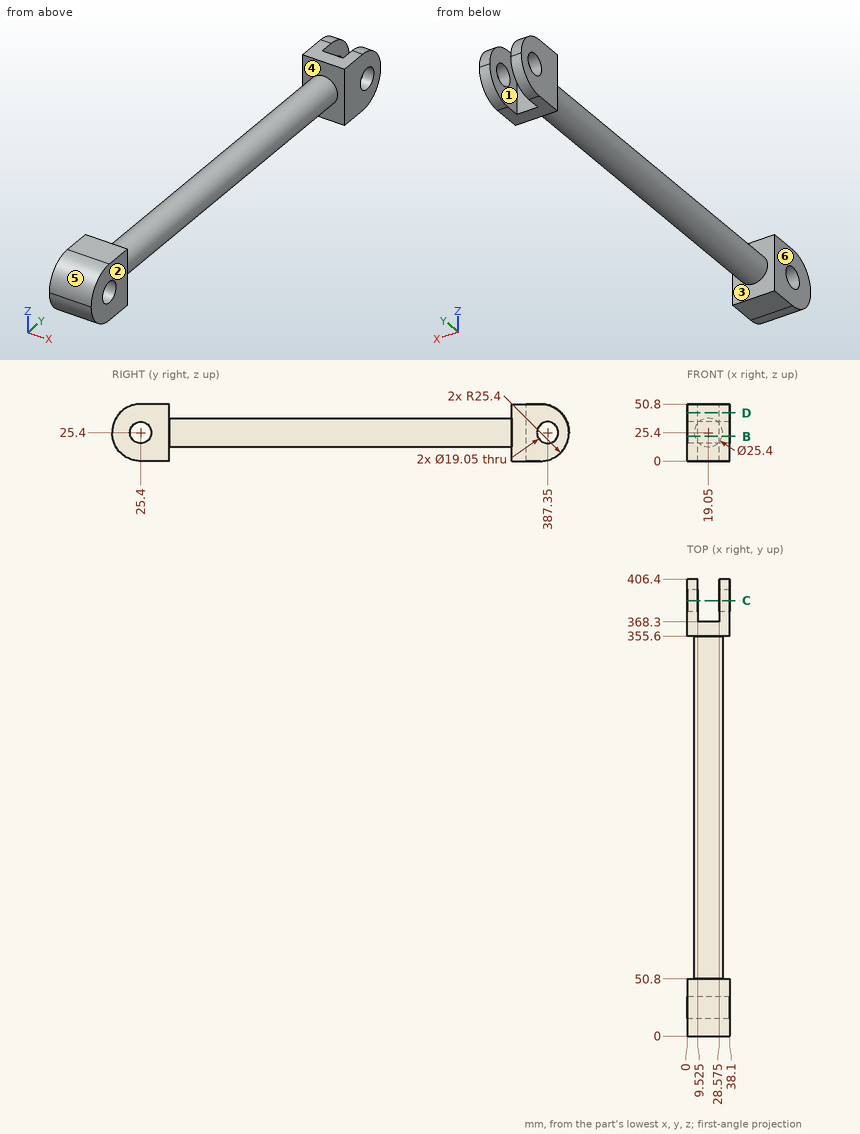
Here's the drawing with two shaded views (mm, measured from the low corner). I have some questions. A direction names the side the tool comes from. Give positions to 0.01 mm unless a question says otherwise; leave off trailing zeros. Order: outer loops, then holes, each group sorted by start corner. A loop starts at its lowest first (then second) coordinate and runs counter-clockwise, first axis right, second up. Notation, with made-up numbers: (-4.75, 40) -> (3.25, 40) arc R19 cw to (3.25, 76) -> close; hole circle Ø9 at (28.25, -35). An arc over 180 degrees is marked (long way). Use a Markdown table: item, result. Add a question column.
Item 1: Imagine slicing it at B-B on z = 22. Please give me the cut outline in (x, y) (1 decimal), plus the area to 3 significant figures.
Item 2: Will these pins go through, and if not, where does the flat tip stop? pin 1 (1.5 mm diameter, centred on y = 272.5, z = 14.5, fed in from +X); pin 2 (15 mm diameter, centred on x = 23, z = 34, fed in from +Y); pin 3 (1.5 mm diameter, centred on x = 27.5, z = 45.5, fed in from +Y).
Item 3: I need wall thicknesses on line 1 (Y direction, x = 7, z = 25); line 2 (Z direction, x = 19.5, y = 25.4) (3 decimals); line 3 (Y direction, x = 21, z = 25). Which ranges of each line are inside material? Lowest first, please.
Item 4: If we mould it in two halves opening along Y, with no side actions, what happens to the marked faces 4, 5 and 6? For each: pulls with the +Y half, pulls with the -Y half, needs draft (parallel to the pull), parting line crosses it, or undercut.
Item 5: Imagine slicing it at D-D on z = 43. Please give me the cut outline in (x, y) (3 decimals), plus the area to 3 significant figures.
Item 6: Imagine slicing it at C-C on y = 387.35. Please give me the cut outline in (x, z) (3 decimals), plus the area to 3 significant figures.
Item 7: For the marked faces 1, 2 and 3, which set-ups out of +Z, -Z, +X, -X, +Y, -Y let a thin tool reach every point of the face, with its end or its side?
Data:
| question | item | result |
|---|---|---|
| 1 | outline | (0, 0.2) -> (38.1, 0.2) -> (38.1, 16.5) -> (0, 16.5) -> close; (0, 34.3) -> (38.1, 34.3) -> (38.1, 50.8) -> (31.3, 50.8) -> (31.3, 355.6) -> (38.1, 355.6) -> (38.1, 378.5) -> (28.6, 378.5) -> (28.6, 368.3) -> (9.5, 368.3) -> (9.5, 378.5) -> (0, 378.5) -> (0, 355.6) -> (6.8, 355.6) -> (6.8, 50.8) -> (0, 50.8) -> close; (0, 396.2) -> (9.5, 396.2) -> (9.5, 406.2) -> (0, 406.2) -> close; (28.6, 396.2) -> (38.1, 396.2) -> (38.1, 406.2) -> (28.6, 406.2) -> close |
| 1 | area | 9,570 mm² |
| 2 | pin 1 | stops at x = 26.68 |
| 2 | pin 2 | stops at y = 406.15 |
| 2 | pin 3 | stops at y = 368.3 |
| 3 | line 1 | y = 0 to 15.88, 34.92 to 377.83, 396.87 to 406.4 |
| 3 | line 2 | z = 0 to 15.875, 34.925 to 50.8 |
| 3 | line 3 | y = 0 to 15.88, 34.92 to 368.3 |
| 4 | face 4 | undercut |
| 4 | face 5 | pulls with the -Y half |
| 4 | face 6 | needs draft |
| 5 | outline | (0, 7.086) -> (38.1, 7.086) -> (38.1, 50.8) -> (0, 50.8) -> close; (0, 355.6) -> (38.1, 355.6) -> (38.1, 399.314) -> (28.575, 399.314) -> (28.575, 368.3) -> (9.525, 368.3) -> (9.525, 399.314) -> (0, 399.314) -> close |
| 5 | area | 2,740 mm² |
| 6 | outline | (0, 0.807) -> (9.525, 0.807) -> (9.525, 15.875) -> (0, 15.875) -> close; (0, 34.925) -> (9.525, 34.925) -> (9.525, 49.993) -> (0, 49.993) -> close; (28.575, 0.807) -> (38.1, 0.807) -> (38.1, 15.875) -> (28.575, 15.875) -> close; (28.575, 34.925) -> (38.1, 34.925) -> (38.1, 49.993) -> (28.575, 49.993) -> close |
| 6 | area | 574 mm² |
| 7 | face 1 | +Z, -Z, +Y |
| 7 | face 2 | +Z, -Z, +X, +Y, -Y |
| 7 | face 3 | none |
